Autodesk Inventor part; units mm, degrees
ref_plane "Work Plane1" through (1.525, 0, 0) normal (0, 0, 1) x (1, 0, 0)
ref_plane "YZ Plane" through (0, 0, 0) normal (1, 0, 0) x (0, 1, 0)
ref_plane "XZ Plane" through (0, 0, 0) normal (0, 1, 0) x (-1, 0, 0)
sketch "Sketch1" plane through (0, 0, 0) normal (0, 0, 1) x (1, 0, 0)
  line L0 (0, 3.5) -> (22, 3.5)
  line L1 (22, 3.5) -> (22, 0)
  line L2 (22, 0) -> (0, 0)
  line L3 (-4.4, 0) -> (26.4, 0)
  line L4 (0, -0.7) -> (0, 4.2)
  line L5 (0, 3.5) -> (0, 0)
  dimension "d2" = 7
  dimension "d59" = 22
revolve "Body" add sketch "Sketch1" angle 360 about axis through (22, 0, 0) along (-1, 0, 0)
sketch "Sketch2" plane through (0, 0, 0) normal (-1, 0, 0) x (0, 0, 1)
  line L0 (0, 6.3509) -> (5.5, 3.1754)
  line L1 (5.5, 3.1754) -> (5.5, -3.1754)
  line L2 (5.5, -3.1754) -> (0, -6.3509)
  line L3 (0, -6.3509) -> (-5.5, -3.1754)
  line L4 (-5.5, -3.1754) -> (-5.5, 3.1754)
  line L5 (-5.5, 3.1754) -> (0, 6.3509)
  line L6 (-7.7, 0) -> (7.7, 0)
  line L7 (0, 8.8912) -> (0, -8.8912)
  point P0 (0, 0)
  point P1 (0, 0)
  dimension "d11" = 11
extrude "Head" add sketch "Sketch2" along normal blind 4.5
sketch "Sketch4" plane through (0, 0, 0) normal (0, 0, 1) x (1, 0, 0)
  line L0 (-3.8649, 6.6) -> (-4.5, 5.5)
  line L1 (-1.1, 0) -> (-0.234, 0)
  line L2 (-5.3532, 0) -> (0.6192, 0)
  line L3 (-4.5, 6.6) -> (-3.8649, 6.6)
  line L4 (-4.5, 5.5) -> (-4.5, 6.6)
  line L5 (0, 7.92) -> (0, -1.32)
  dimension "d65" = 11
  dimension "d67" = 30
  dimension "d68" = 13.2
  dimension "d69" = 4.5
revolve "Chamfer1" cut sketch "Sketch4" angle 360 about axis through (-1.1, 0, 0) along (1, 0, 0)
thread "Thread"
chamfer "Chamfer2" distance 0.6135 distance2 0.6136 1 edges at (22, -3.5, 0) measured on face at (22, 0.6242, -1.2774)
fillet "Fillet2" radius 0.3 1 edges at (0, -3.5, 0)
ref_plane "Work Plane1" through (1.525, 0, 0) normal (0, 0, 1) x (1, 0, 0)
equation "\"d2\" = GD"
equation "\"d59\" = NLG"
equation "\"d11\" = SW"
equation "\"d3\" = KOH"
equation "\"d71\" = RR"
equation "\"d15\" = GEL"
equation "\"d6\" = -0.5 * SPD + 0.5 * GD"
equation "\"d65\" = SW"
equation "\"d67\" = ANG1"
equation "\"d68\" = 1.2 * SW"
equation "\"d69\" = KOH"
equation "\"NLG\" = 22"
equation "\"GD\" = NND"
equation "\"BDM\" = NND"
equation "\"KOH\" = 4.5"
equation "\"GEL\" = 13"
equation "\"SW\" = 11"
equation "\"SW0\" = 11"
equation "\"SPD\" = NND - 1.2269 * PTC"
equation "\"SD2\" = NND"
equation "\"SD\" = 0"
equation "\"ANG1\" = 30deg"
equation "\"GAL\" = 0.61345 * PTC"
equation "\"GUL\" = 0.61345 * PTC"
equation "\"RR\" = 0.3"
equation "\"RR1\" = 0.1"
equation "\"GD1\" = THREADDIA - 1.2269 * PTC"
equation "\"THREADDIA\" = 7"
equation "\"TOA\" = 30deg"
equation "\"FAWI\" = 60deg"
equation "\"PTC\" = 1"
equation "\"NND\" = 7"
equation "\"E0\" = 1.155 * SW"
properties part number "CSN 02 1201 - M7 x 22" material "Steel, Mild"
Verification items for the finished model (mm, model axes). A direction names the side the tool comes from. Round coordinates to 2 decimals unless told otherwise and drop trailing zeros. Loops run counter-clockwise (first coordinate to the right, second up) from the corner with the lowest first, then second, coordinate; pieces in that order, holes last. Notation, with made-up numbers: (-28.75, 69.5) - (-2.75, 69.5) arc R30 ccw to (-2.75, 98.5) - close; hole circle Ø4 at (65, 52.25). An arc over 180 degrees is marked (long way). Use one line per item in the form item = value.
1. Scan lines: probe 1 along Y at (x, z) = (-1, 2.75); probe 2 along X at (y, z) = (1.75, -4.5); probe 3 along Y at (x, z) = (17.5, 3). Record each from-to range of solid material in increasing order.
A:
probe_1 = -4.76 to 4.76
probe_2 = -4.5 to 0
probe_3 = -1.8 to 1.8
2. Gauge pin test, flat ends, axial feed: pin 1 Ø3 at (x, y) = (11, 4.5) entering from -Z; pin 2 Ø1.5 at (x, z) = (3.5, 1) entering from +Y; pin 3 Ø1.5 at (x, y) = (9, 3) entering from +Z. Record the tip position at first contact, or that the pin passes through.
A:
pin_1 = -1.8
pin_2 = 3.49
pin_3 = 2.68
3. Access from +Z, -Z, +X, -X, +Y, -Y to the whole of each face (thin tool, end or side, straight path). Record for faces 1 (the conical face through (-4.38, 5.71, -0.01)), 2 (the flat face through (0, -1, -4)).
A:
face_1 = -X, +Y
face_2 = +X
4. Section check A-A on x = 19.75. Record the cut outline in (y, z).
A:
outline = circle Ø7 at (0, 0)
